from build123d import *

# Parameters (mm, degrees)
SKETCH1_W           = 508
SKETCH1_H           = 190.5
BOSS_EXTRUDE1_DEPTH = 6.35
SKETCH2_W           = 508
SKETCH2_H           = 190.5
SKETCH2_W_2         = 495.3
SKETCH2_H_2         = 177.8
BOSS_EXTRUDE2_DEPTH = 298.45
SKETCH3_W           = 6.35
SKETCH3_H           = 16.933333333
SKETCH3_H_2         = 16.933333334
CUT_EXTRUDE1_DEPTH  = 12.7
SKETCH4_W           = 6.35
SKETCH4_H           = 15.875
CUT_EXTRUDE2_DEPTH  = 6.35
SKETCH6_W           = 514.801062296
SKETCH6_H           = 254.881465808
CUT_EXTRUDE5_DEPTH  = 305.8
SKETCH5_W           = 6.35
SKETCH5_H           = 16.933333333
SKETCH5_H_2         = 16.933333334
CUT_EXTRUDE6_DEPTH  = 6.35
SKETCH7_W           = 6.35
SKETCH7_H           = 12.7
CUT_EXTRUDE7_DEPTH  = 7.35


with BuildPart() as part:
    # Sketch1 → Boss-Extrude1 (new body)
    with BuildSketch(Plane(origin=(0, 0, 0), x_dir=(1, 0, 0), z_dir=(0, 1, 0))):
        Rectangle(SKETCH1_W, SKETCH1_H)
    extrude(amount=BOSS_EXTRUDE1_DEPTH)

    # Sketch2 → Boss-Extrude2 (add)
    with BuildSketch(Plane(origin=(0, 6.35, 0), x_dir=(1, 0, 0), z_dir=(0, 1, 0))):
        Rectangle(SKETCH2_W, SKETCH2_H)
        Rectangle(SKETCH2_W_2, SKETCH2_H_2, mode=Mode.SUBTRACT)
    extrude(amount=BOSS_EXTRUDE2_DEPTH)

    # Sketch3 → Cut-Extrude1 (cut)
    with BuildSketch(Plane.XY.offset(95.25)):
        with BuildLine():
            Line((-3.302, 283.21), (-3.302, 6.35))
            Line((-3.302, 6.35), (3.302, 6.35))
            Line((3.302, 6.35), (3.302, 292.354))
            Line((3.302, 292.354), (-16.256, 292.354))
            Line((-16.256, 292.354), (-16.256, 285.75))
            Line((-16.256, 285.75), (-5.842, 285.75))
            ThreePointArc((-5.842, 285.75), (-4.045948776, 285.006051224), (-3.302, 283.21))
        make_face()
        with Locations((12.827, 80.433333334)):
            Rectangle(SKETCH3_W, SKETCH3_H)
        with Locations((12.827, 50.8)):
            Rectangle(SKETCH3_W, SKETCH3_H_2)
        with Locations((12.827, 21.166666667)):
            Rectangle(SKETCH3_W, SKETCH3_H)
    extrude(amount=-CUT_EXTRUDE1_DEPTH, mode=Mode.SUBTRACT)

    # Sketch4 → Cut-Extrude2 (cut)
    with BuildSketch(Plane.XY.offset(-88.9)):
        with Locations((-19.431, 284.1625)):
            Rectangle(SKETCH4_W, SKETCH4_H)
        with Locations((-19.431, 255.5875)):
            Rectangle(SKETCH4_W, SKETCH4_H)
        with Locations((-19.431, 227.0125)):
            Rectangle(SKETCH4_W, SKETCH4_H)
        with Locations((-19.431, 198.4375)):
            Rectangle(SKETCH4_W, SKETCH4_H)
        with Locations((-19.431, 169.8625)):
            Rectangle(SKETCH4_W, SKETCH4_H)
        with Locations((-19.431, 141.2875)):
            Rectangle(SKETCH4_W, SKETCH4_H)
        with Locations((-19.431, 112.7125)):
            Rectangle(SKETCH4_W, SKETCH4_H)
        with Locations((-19.431, 84.1375)):
            Rectangle(SKETCH4_W, SKETCH4_H)
        with Locations((-19.431, 55.5625)):
            Rectangle(SKETCH4_W, SKETCH4_H)
        with Locations((-19.431, 26.9875)):
            Rectangle(SKETCH4_W, SKETCH4_H)
    cut_extrude2 = extrude(amount=-CUT_EXTRUDE2_DEPTH, mode=Mode.SUBTRACT)

    # Mirror1: Cut-Extrude2 across plane
    add(cut_extrude2.mirror(Plane.ZY.offset(6.477)), mode=Mode.SUBTRACT)

    # Sketch6 → Cut-Extrude5 (cut, through all)
    with BuildSketch(Plane(origin=(0, 0, 0), x_dir=(1, 0, 0), z_dir=(0, 1, 0))):
        with Locations((9.750531148, -10.000845247)):
            Rectangle(SKETCH6_W, SKETCH6_H)
    extrude(amount=CUT_EXTRUDE5_DEPTH, mode=Mode.SUBTRACT)

    # Sketch5 → Cut-Extrude6 (cut)
    with BuildSketch(Plane(origin=(0, 0, 0), x_dir=(-1, 0, 0), z_dir=(0, -1, 0))):
        with Locations((250.825, -74.083333334)):
            Rectangle(SKETCH5_W, SKETCH5_H)
        with Locations((250.825, -44.45)):
            Rectangle(SKETCH5_W, SKETCH5_H_2)
        with Locations((250.825, -14.816666667)):
            Rectangle(SKETCH5_W, SKETCH5_H)
        with Locations((250.825, 14.816666667)):
            Rectangle(SKETCH5_W, SKETCH5_H)
        with Locations((250.825, 44.45)):
            Rectangle(SKETCH5_W, SKETCH5_H_2)
        with Locations((250.825, 74.083333334)):
            Rectangle(SKETCH5_W, SKETCH5_H)
    extrude(amount=-CUT_EXTRUDE6_DEPTH, mode=Mode.SUBTRACT)

    # Sketch7 → Cut-Extrude7 (cut, through all)
    with BuildSketch(Plane.ZY.offset(254)):
        with Locations((-92.075, 32.904545455)):
            Rectangle(SKETCH7_W, SKETCH7_H)
        with Locations((-92.075, 6.35)):
            Rectangle(SKETCH7_W, SKETCH7_H)
        with Locations((-92.075, 59.459090909)):
            Rectangle(SKETCH7_W, SKETCH7_H)
        with Locations((-92.075, 86.013636364)):
            Rectangle(SKETCH7_W, SKETCH7_H)
        with Locations((-92.075, 112.568181818)):
            Rectangle(SKETCH7_W, SKETCH7_H)
        with Locations((-92.075, 139.122727273)):
            Rectangle(SKETCH7_W, SKETCH7_H)
        with Locations((-92.075, 165.677272727)):
            Rectangle(SKETCH7_W, SKETCH7_H)
        with Locations((-92.075, 192.231818182)):
            Rectangle(SKETCH7_W, SKETCH7_H)
        with Locations((-92.075, 218.786363636)):
            Rectangle(SKETCH7_W, SKETCH7_H)
        with Locations((-92.075, 245.340909091)):
            Rectangle(SKETCH7_W, SKETCH7_H)
        with Locations((-92.075, 271.895454545)):
            Rectangle(SKETCH7_W, SKETCH7_H)
        with Locations((-92.075, 298.45)):
            Rectangle(SKETCH7_W, SKETCH7_H)
        with Locations((92.075, 298.45)):
            Rectangle(SKETCH7_W, SKETCH7_H)
        with Locations((92.075, 271.895454545)):
            Rectangle(SKETCH7_W, SKETCH7_H)
        with Locations((92.075, 245.340909091)):
            Rectangle(SKETCH7_W, SKETCH7_H)
        with Locations((92.075, 218.786363636)):
            Rectangle(SKETCH7_W, SKETCH7_H)
        with Locations((92.075, 192.231818182)):
            Rectangle(SKETCH7_W, SKETCH7_H)
        with Locations((92.075, 165.677272727)):
            Rectangle(SKETCH7_W, SKETCH7_H)
        with Locations((92.075, 139.122727273)):
            Rectangle(SKETCH7_W, SKETCH7_H)
        with Locations((92.075, 112.568181818)):
            Rectangle(SKETCH7_W, SKETCH7_H)
        with Locations((92.075, 86.013636364)):
            Rectangle(SKETCH7_W, SKETCH7_H)
        with Locations((92.075, 59.459090909)):
            Rectangle(SKETCH7_W, SKETCH7_H)
        with Locations((92.075, 32.904545455)):
            Rectangle(SKETCH7_W, SKETCH7_H)
        with Locations((92.075, 6.35)):
            Rectangle(SKETCH7_W, SKETCH7_H)
    extrude(amount=-CUT_EXTRUDE7_DEPTH, mode=Mode.SUBTRACT)


solid = part.part
The model under review builds one solid part; all positions refer to its coordinate system, in mm. A direction names the side the tool comes from. Give positions to 0.01 mm unless a question says otherwise; leave off trailing zeros. Order: outer loops, then holes, each group sorted by start corner. A loop starts at its lowest first (then second) coordinate and runs counter-clockwise, first axis right, second up. Notation, with made-up numbers: M 51.25,46.5 L 102.25,46.5 A9 cw 102.25,57.5 Z; hole C 72,36.25 d5. An arc over 180 degrees is marked long. Use one line per item in the form item = value. Start each with the question number.
Item 1: Insertion check: pin 1 Ø3 at (x, z) = (-251.5, 93) entering from +Y; pin 2 Ø3 at (x, y) = (-251, 3) entering from +Z; pin 3 Ø1.9 at (x, z) = (-250, -92) entering from -Y. Each pin has a flat end and moves straight along its axis. Give the tip position at first contact, or say it passes through.
Item 2: For faces 1 (the flat face through (-251, 132.773, -92)), 2 (the flat face through (-251, 118.918, 92)), 3 (the flat face through (-247.65, 150, 1)), list the 3-axis set-ups (+Z, -Z, +X, -X, +Y, -Y) from which the entire face can be reached by the end or side of a thin tool; tool diameter is ignored.
Item 3: We need section B-B on y = 58. Give the boundary of the cut face in (x, z), plus the area to 3 significant figures.
Item 4: The part is to be moulded in two halves that separate along Y. For faces 4 (the flat face through (-251, 6.35, 74)), 5 (the flat face through (-251, 152, -95.25)), 6 (the flat face through (-251, 166, -88.9)), say which applies: pulls with the +Y half, pulls with the -Y half, needs draft (parallel to the pull), parting line crosses it, or undercut.
Item 5: We need section A-A on z = 79.5. Give the boundary of the cut face in (x, y).
Item 6: To check wall thickness, follow line 1 along Y through (x, z) = (-250, 37); line 2 along Z through (x, y) = (-251.5, 217). State the ranges of each line that lie inside material, in increasing order. Write a range as from..to.
Completed:
q1.pin_1 = 292.1
q1.pin_2 = 88.9
q1.pin_3 = 12.7
q2.face_1 = -Z, +X, -X
q2.face_2 = +Z, +X, -X
q2.face_3 = +Z, -Z, +X, +Y, -Y
q3.outline = M -254,-88.9 L -247.65,-88.9 L -247.65,88.9 L -254,88.9 Z
q3.area = 1,130 mm²
q4.face_4 = pulls with the -Y half
q4.face_5 = needs draft
q4.face_6 = undercut
q5.outline = M -254,6.35 L -247.65,6.35 L -247.65,304.8 L -254,304.8 Z
q6.line_1 = 6.35..304.8
q6.line_2 = -88.9..88.9
